Build history of the part. All positions in model axes, mm. Give positions to 0.01 mm unless a question says otherwise; leave off trailing zeros. Loops run counter-clockwise (first coordinate to the right, second up) from the corner with the lowest first, then second, coordinate; pieces in that order, holes last. Notation, with made-up numbers: M 52,59 L 61,59 A34 ccw 61,95 Z; hole C 58,2 d3. An arc over 180 degrees is marked long. Answer in a Markdown table with one row per item. Add a question column.
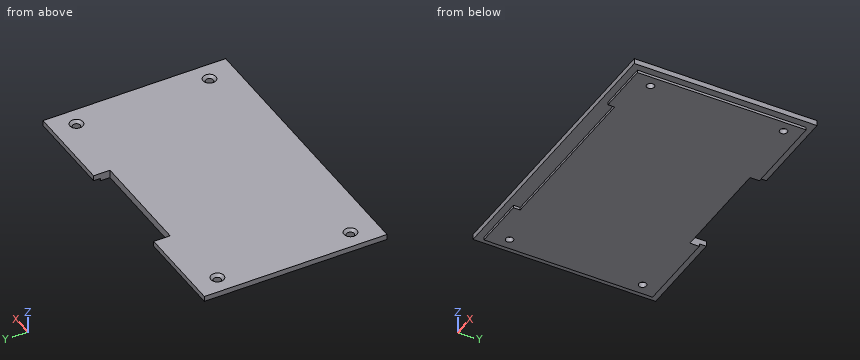
Autodesk Inventor part; units mm, degrees
ref_plane "YZ Plane" through (0, 0, 0) normal (1, 0, 0) x (0, 1, 0)
ref_plane "XZ Plane" through (0, 0, 0) normal (0, 1, 0) x (-1, 0, 0)
ref_plane "XY Plane" through (0, 0, 0) normal (0, 0, 1) x (1, 0, 0)
sketch "Sketch1" plane through (0, 0, 0) normal (0, 0, 1) x (1, 0, 0)
  line L0 (107.6, 68) -> (107.6, 0)
  line L1 (107.6, 0) -> (0, 0)
  line L2 (0, 0) -> (0, 68)
  line L3 (0, 68) -> (33.75, 68)
  line L4 (33.75, 68) -> (33.75, 61.9)
  line L5 (33.75, 61.9) -> (73.85, 61.9)
  line L6 (73.85, 61.9) -> (73.85, 68)
  line L7 (73.85, 68) -> (107.6, 68)
  line L8 (53.8, 0) -> (53.8, -26.1159) construction
  line L9 (53.8, 61.9) -> (53.8, 35.6829) construction
  dimension "d37" = 40.1
  dimension "d38" = 107.6
  dimension "d39" = 68
  dimension "d64" = 6.1
extrude "Extrusion1" add sketch "Sketch1" along normal blind 3
sketch "Sketch4" plane through (0, 0, 0) normal (0, 0, -1) x (-1, 0, 0)
  line L0 (-33.75, 68) -> (0, 68)
  line L1 (-33.75, 61.9) -> (-33.75, 68)
  line L2 (-73.85, 61.9) -> (-33.75, 61.9)
  line L3 (-73.85, 68) -> (-73.85, 61.9)
  line L4 (-107.6, 68) -> (-73.85, 68)
  line L5 (-107.6, 0) -> (-107.6, 68)
  line L6 (0, 0) -> (-107.6, 0)
  line L7 (0, 68) -> (0, 0)
  line L8 (-71.25, 65.4) -> (-71.25, 63.4)
  line L9 (-71.25, 63.4) -> (-36.35, 63.4)
  line L10 (-36.35, 63.4) -> (-36.35, 65.4)
  line L11 (-36.35, 65.4) -> (-2.6, 65.4)
  line L12 (-71.25, 65.4) -> (-105, 65.4)
  line L13 (-105, 65.4) -> (-105, 2.6)
  line L14 (-2.6, 2.6) -> (-2.6, 65.4)
  line L15 (-105, 2.6) -> (-85.29, 2.6)
  line L16 (-85.29, 2.6) -> (-85.29, 5.1)
  line L17 (-85.29, 5.1) -> (-22.31, 5.1)
  line L18 (-22.31, 5.1) -> (-22.31, 2.6)
  line L19 (-22.31, 2.6) -> (-2.6, 2.6)
  line L20 (-53.8, 0) -> (-53.8, 2.6) construction
  line L21 (-53.8, 5.1) -> (-53.8, 2.6) construction
  dimension "d42" = 2.6
  dimension "d43" = 2.6
  dimension "d44" = 2.6
  dimension "d45" = 2.6
  dimension "d46" = 2.6
  dimension "d48" = 2.6
  dimension "d49" = 5.1
  dimension "d50" = 2.6
  dimension "d51" = 2.6
  dimension "d52" = 62.98
  dimension "d65" = 2
extrude "Extrusion4" cut sketch "Sketch4" against normal blind 1 contours L0 L7 L6 L5 L4 L3 L12 L13 L15 L16 L17 L18 L19 L14 L11 L1
sketch "Sketch5" plane through (0, 0, 3) normal (0, 0, 1) x (1, 0, 0)
  circle A0 centre (6.8128, 9.8088) radius 1.5
  circle A1 centre (6.81, 59.3388) radius 1.5
  circle A2 centre (100.7928, 9.8142) radius 1.5
  circle A3 centre (100.79, 59.3442) radius 1.5
  line L0 (104.603, 6.0044) -> (3.003, 5.9986)
  line L1 (104.5998, 63.1544) -> (104.603, 6.0044)
  line L2 (2.9998, 63.1486) -> (104.5998, 63.1544)
  line L3 (3.003, 5.9986) -> (2.9998, 63.1486)
  circle A4 centre (6.81, 59.3388) radius 1.4
  circle A5 centre (6.8128, 9.8088) radius 1.4
  circle A6 centre (100.7928, 9.8142) radius 1.4
  circle A7 centre (100.79, 59.3442) radius 1.4
  point P0 (0, 0)
  dimension "d55" = 2.8
  dimension "d56" = 2.8
  dimension "d57" = 2.8
  dimension "d58" = 2.8
extrude "Extrusion5" cut sketch "Sketch5" against normal blind 4 contours A4 | A5 | A6 | A7
chamfer "Chamfer3" distance 1 angle 45 4 edges at (5.41, 59.3388, 3) (5.4128, 9.8088, 3) (99.39, 59.3442, 3) (99.3928, 9.8142, 3)
properties part number "Enclosure-Backplate01"
(1) Wall check: line 1 (Y direction, x = 100.79, z = 1.5); line 2 (Y direction, x = 100.79, z = 0.95); line 3 (X direction, y = 59, z = 1.05). Give the ranges that are in metal, low to high.
(2) Pin check, flat tips, straight feed: pin 1 (0.8 mm diameter, centred on y = 35.5, z = 0.5, fed in from +X); pin 2 (0.5 mm diameter, centred on x = 64, z = 0.5, fed in from -Y); pin 3 (0.5 mm diameter, centred on x = 87, z = 0.5, fed in from +Y). Stop position of each tip, or through.
(3) Slice it at A-A, the plane y = 23. Give the cut face in (x, z), then the cut area to 3 significant figures.
(4) Slice it at B-B, the plane x = 76. Give the cut face in (y, z).
(5) Slice it at D-D, the plane x = 60.5. Give the cut face in (y, z).
(6) Slice it at C-C, the plane x = 6.81. State how many separate pieces and enclosed holes the cut face has, then the cut area to 3 significant figures.
Solution:
| question | item | result |
|---|---|---|
| 1 | line 1 | 0 to 8.41, 11.21 to 57.94, 60.74 to 68 |
| 1 | line 2 | 2.6 to 8.41, 11.21 to 57.94, 60.74 to 65.4 |
| 1 | line 3 | 0 to 5.45, 8.17 to 99.43, 102.15 to 107.6 |
| 2 | pin 1 | x = 105 |
| 2 | pin 2 | y = 5.1 |
| 2 | pin 3 | y = 65.4 |
| 3 | outline | M 0,1 L 2.6,1 L 2.6,0 L 105,0 L 105,1 L 107.6,1 L 107.6,3 L 0,3 Z |
| 3 | area | 318 mm^2 |
| 4 | outline | M 0,1 L 5.1,1 L 5.1,0 L 65.4,0 L 65.4,1 L 68,1 L 68,3 L 0,3 Z |
| 5 | outline | M 0,1 L 5.1,1 L 5.1,0 L 61.9,0 L 61.9,3 L 0,3 Z |
| 6 | separate pieces | 3 |
| 6 | enclosed holes | 0 |
| 6 | area | 180 mm^2 |
